Verification items for the finished model (mm, model axes). A direction names the side the tool comes from. Coordinates: 2 decimals unless noted, no trailing zeros. Write each loop counter-clockwise with the first axis right and the second up, starting at its lowest first coordinate (ties: lowest second). Pieces come first, ordered by that corner, then holes. Notation, with made-up numbers: (-25.5, 39.5) -> (-5.5, 39.5) arc R26 cw to (-5.5, 76.5) -> close; hole circle Ø2 at (-22.75, -4). An arc over 180 degrees is marked (long way). Use CSV: the item, a comma, the result in double quotes.
```python
from build123d import *

# Parameters (mm, degrees)
ESQUISSE1_W                         = 10
ESQUISSE1_H                         = 18
BOSS_EXTRU_1_DEPTH                  = 1
ESQUISSE2_W                         = 8
ESQUISSE2_H                         = 13.4
BOSS_EXTRU_2_DEPTH                  = 1.7
ESQUISSE3_W                         = 7
ESQUISSE3_H                         = 1.7
BOSS_EXTRU_3_DEPTH                  = 2.2
DIAM_TRE_DU_PER_AGE_0_9_0_9_1_D     = 0.9
DIAM_TRE_DU_PER_AGE_0_9_0_9_1_DEPTH = 3.2


with BuildPart() as part:
    # Esquisse1 → Boss.-Extru.1 (new body)
    with BuildSketch(Plane(origin=(0, 1, 0), x_dir=(1, 0, 0), z_dir=(0, 1, 0))):
        Rectangle(ESQUISSE1_W, ESQUISSE1_H)
    extrude(amount=-BOSS_EXTRU_1_DEPTH)

    # Esquisse2 → Boss.-Extru.2 (add)
    with BuildSketch(Plane(origin=(0, 1, 0), x_dir=(-1, 0, 0), z_dir=(0, 1, 0))):
        with Locations((0, 1.3)):
            Rectangle(ESQUISSE2_W, ESQUISSE2_H)
    extrude(amount=BOSS_EXTRU_2_DEPTH)

    # Esquisse3 → Boss.-Extru.3 (add)
    with BuildSketch(Plane(origin=(0, 1, 0), x_dir=(-1, 0, 0), z_dir=(0, 1, 0))):
        with Locations((0.79, -7.48)):
            Rectangle(ESQUISSE3_W, ESQUISSE3_H)
    extrude(amount=BOSS_EXTRU_3_DEPTH)

    # Diamètre du perçage Ø0.9 (0.9)1
    with Locations(Plane(origin=(0, 0, 0), x_dir=(-1, 0, 0), z_dir=(0, -1, 0))):
        with Locations((-4, 7.25)):
            Hole(DIAM_TRE_DU_PER_AGE_0_9_0_9_1_D / 2, depth=DIAM_TRE_DU_PER_AGE_0_9_0_9_1_DEPTH)


solid = part.part
```
1) Set-up check for faces 5 (the flat face through (0, 2.7, 1)), 6 (the flat face through (-1, 2, -6.63)), 7 (the flat face through (-4, 2, 1)): record each of +Z, -Z, +X, -X, +Y, -Y from which the full face is reachable in a straight line by a thin tool's end or side.
Return value:
face 5,"+Z, +X, -X, +Y"
face 6,"+X, -X, +Y"
face 7,"+Z, -X, +Y"
2) Cross-section at D-D (x = -2.75). Record the boundary of the cut face in (y, z).
Return value:
outline,"(0, -9) -> (1, -9) -> (1, -8.33) -> (3.2, -8.33) -> (3.2, -6.63) -> (1, -6.63) -> (1, -5.4) -> (2.7, -5.4) -> (2.7, 8) -> (1, 8) -> (1, 9) -> (0, 9) -> close"
3) Cross-section at A-A (z = -7.25). Record the boundary of the cut face in (x, y), plus the area to 3 significant figures.
Return value:
outline,"(-5, 0) -> (3.55, 0) -> (3.55, 1) -> (2.71, 1) -> (2.71, 3.2) -> (-4.29, 3.2) -> (-4.29, 1) -> (-5, 1) -> close; (4.45, 0) -> (5, 0) -> (5, 1) -> (4.45, 1) -> close"
area,"24.5 mm2"
4) Scan lines: L1, parallel to X at y = 0.45, z = -7.25; L2, parallel to Z at x = 4, y = 0.8; L3, parallel to Z at x = -3, y = 1.2. Record each from-to range of solid material in increasing order.
Return value:
L1,"-5 to 3.55, 4.45 to 5"
L2,"-9 to -7.7, -6.8 to 9"
L3,"-8.33 to -6.63, -5.4 to 8"
5) Mould release check, pull along X, two halves, no side actions. Record for faces 1 (the flat face through (2.71, 2, -7)), 2 (the cylindrical face through (3.941, 0.507, -7.696)), 3 (the flat face through (-4.29, 2, -7)), 4 (the flat face through (0, 2, -5.4)): released by +X, released by -X, zero draft, split by the parting line, or undercut.
Return value:
face 1,"released by +X"
face 2,"undercut"
face 3,"released by -X"
face 4,"zero draft"
6) Gauge pin test, flat ends, axial feed: pin 1 (1.4 mm diameter, centred on y = 2.5, z = -7.5, fed in from +X); pin 2 (6 mm diameter, centred on x = -0.5, z = -4, fed in from -Y); pin 3 (0.5 mm diameter, centred on y = 2, z = 1, fed in from -X); pin 4 (1 mm diameter, centred on x = 2, y = 2, fed in from -Z). Record the tip position at first contact, or that the pin passes through.
Return value:
pin 1,"x = 2.71"
pin 2,"y = 0"
pin 3,"x = -4"
pin 4,"z = -8.33"
7) Cross-section at C-C (z = -4.5). Record the boundary of the cut face in (x, y), plus the area to 3 significant figures.
Return value:
outline,"(-5, 0) -> (5, 0) -> (5, 1) -> (4, 1) -> (4, 2.7) -> (-4, 2.7) -> (-4, 1) -> (-5, 1) -> close"
area,"23.6 mm2"
8) Cross-section at B-B (y = 2.2). Record the boundary of the cut face in (x, z).
Return value:
outline,"(-4.29, -8.33) -> (2.71, -8.33) -> (2.71, -6.63) -> (-4.29, -6.63) -> close; (-4, -5.4) -> (4, -5.4) -> (4, 8) -> (-4, 8) -> close"
